from build123d import *

# Parameters (mm, degrees)
F0_W     = 130.542636
F0_H     = 127.233949
F1_DEPTH = 9.906
F2_W     = 19.73008
F2_H     = 21.76354
F2_W_2   = 20.498451
F2_H_2   = 26.257996
F2_W_3   = 20.644247
F2_H_3   = 18.675257
F2_W_4   = 19.04821
F2_H_4   = 20.091395
F3_DEPTH = 187.706
F4_W     = 124.663566
F4_H     = 8.92711
F5_DEPTH = 177.8
F6_W     = 8.759178
F6_H     = 129.845535
F6_W_2   = 11.253112
F6_H_2   = 123.803681
F6_W_3   = 15.531029
F6_H_3   = 116.437322
F7_DEPTH = 25.4


with BuildPart() as f1:
    # F0 (on Top) → F1 (new body)
    with BuildSketch(Plane.XY):
        with Locations((2.255924, 3.91026)):
            Rectangle(F0_W, F0_H)
    extrude(amount=F1_DEPTH)

    # F2 (on face) → F3 (join)
    with BuildSketch(Plane.XY):
        with Locations((50.939338, -43.50264)):
            Rectangle(F2_W, F2_H)
        with Locations((51.323523, 45.077661)):
            Rectangle(F2_W_2, F2_H_2)
        with Locations((-44.336367, 48.86903)):
            Rectangle(F2_W_3, F2_H_3)
        with Locations((-43.538349, -42.666567)):
            Rectangle(F2_W_4, F2_H_4)
    extrude(amount=F3_DEPTH)

    # F4 (on face) → F5 (join)
    with BuildSketch(Plane.XY):
        with Locations((1.841141, 63.281318)):
            Rectangle(F4_W, F4_H)
    extrude(amount=-F5_DEPTH)

    # F6 (on face) → F7 (cut)
    with BuildSketch(Plane.XZ.offset(-58.817763)):
        with Locations((42.374756, -78.830328)):
            Rectangle(F6_W, F6_H)
        with Locations((13.268729, -75.809401)):
            Rectangle(F6_W_2, F6_H_2)
        with Locations((-34.073861, -72.126222)):
            Rectangle(F6_W_3, F6_H_3)
    extrude(amount=-F7_DEPTH, mode=Mode.SUBTRACT)


solid = f1.part
Verification items for the finished model (mm, model axes). A direction names the side the tool comes from. Coordinates: 2 decimals unless noted, no trailing zeros. Loops run counter-clockwise (first coordinate to the right, second up) from the corner with the lowest first, then second, coordinate; pieces in that order, holes last. Notation, with made-up numbers: (73, 77) -> (119, 77) arc R34 cw to (119, 109) -> close; hole circle Ø7 at (68, 16). An arc over 180 degrees is marked (long way). Write each question's results on one line, items separated by ' | '.
Item 1: Gauge pin test, flat ends, axial feed: pin 1 (8 mm diameter, centred on y = 48.5, z = 65.5, fed in from -X); pin 2 (12 mm diameter, centred on x = -5, y = 52.5, fed in from +Z); pin 3 (12 mm diameter, centred on x = 40, z = 81, fed in from -Y). Record the tip position at first contact, or that the pin passes through.
Found:
pin 1: stops at x = -54.66 | pin 2: stops at z = 9.91 | pin 3: stops at y = -54.38
Item 2: Tool access check on faces 1 (the face through (37.995, 63, -80)), 2 (the face through (51, 31.949, 98)), 3 (the face through (61.573, 45, 98)). Record the directions out of +Z, -Z, +X, -X, +Y, -Y that give a thin tool (end or side, any length) a straight path to the whole face; none if there is none.
Found:
face 1: +Y, -Y | face 2: +Z, +X, -X | face 3: +Z, +X, +Y, -Y
Item 3: Section check C-C, the plane z = 132. Enter the section's corners in (x, y), plus the area to 3 significant figures.
Found:
outline: (-54.66, 39.53) -> (-34.01, 39.53) -> (-34.01, 58.21) -> (-54.66, 58.21) -> close; (-53.06, -52.71) -> (-34.01, -52.71) -> (-34.01, -32.62) -> (-53.06, -32.62) -> close; (41.07, -54.38) -> (60.8, -54.38) -> (60.8, -32.62) -> (41.07, -32.62) -> close; (41.07, 31.95) -> (61.57, 31.95) -> (61.57, 58.21) -> (41.07, 58.21) -> close | area: 1,740 mm2
Item 4: Section check A-A, the plane z = -114. Enter the section's corners in (x, y).
Found:
outline: (-60.49, 58.82) -> (-41.84, 58.82) -> (-41.84, 67.74) -> (-60.49, 67.74) -> close; (-26.31, 58.82) -> (7.64, 58.82) -> (7.64, 67.74) -> (-26.31, 67.74) -> close; (18.9, 58.82) -> (38, 58.82) -> (38, 67.74) -> (18.9, 67.74) -> close; (46.75, 58.82) -> (64.17, 58.82) -> (64.17, 67.74) -> (46.75, 67.74) -> close
Item 5: Section check D-D, the plane z = -154. Enter the section's corners in (x, y).
Found:
outline: (-60.49, 58.82) -> (64.17, 58.82) -> (64.17, 67.74) -> (-60.49, 67.74) -> close
Item 6: Material ranges on L1, parallel to X at y = 57.5, z = 76.5; L2, parallel to X at y = -33, z = 173; L3, parallel to Y at x = 27, z = -19.5, recorded low to high.
Found:
L1: x = -54.66 to -34.01, 41.07 to 61.57 | L2: x = -53.06 to -34.01, 41.07 to 60.8 | L3: y = 58.82 to 67.74
Item 7: Mould release check, pull along X, two halves, no side actions. Record for faces 4 (the face through (-26.308, 63, -73)), 5 (the face through (67.527, 3, 5)), 6 (the face through (51, 58.207, 98)): +X half, -X half, draft (parallel to the pull), parting line (faces both ways), or undercut.
Found:
face 4: undercut | face 5: +X half | face 6: draft
Item 8: Section check B-B, the plane y = 52. Enter the section's corners in (x, z).
Found:
outline: (-63.02, 0) -> (67.53, 0) -> (67.53, 9.91) -> (61.57, 9.91) -> (61.57, 187.71) -> (41.07, 187.71) -> (41.07, 9.91) -> (-34.01, 9.91) -> (-34.01, 187.71) -> (-54.66, 187.71) -> (-54.66, 9.91) -> (-63.02, 9.91) -> close
